The model under review builds one solid part; all positions refer to its coordinate system, in mm. A direction names the side the tool comes from. Coordinates: 2 decimals unless noted, no trailing zeros. Loops run counter-clockwise (first coordinate to the right, second up) from the corner with the lowest first, then second, coordinate; pieces in that order, holes last. Notation, with made-up numbers: (36, 81.25) - (69, 81.25) arc R28 ccw to (69, 107.25) - close; hole circle Ø8 at (58.5, -23.75). An arc over 180 degrees is marked (long way). Answer in a Markdown table with one row per item. Add a question column.
(1) We need section C-C on z = 6. Give the number of separate pieces and of enclosed holes in the cut face, plus the area to 3 significant figures.
(2) For line 1 along Y through (x, z) = (-15.5, 3.75); line 2 along Z through (x, y) = (-38, 23); line 3 along X through (y, z) = (8.5, 13.5), list the stretches that pass through material, from the lowest coordinate up.
(3) We need section A-A on x = 38.06. Write out the cut boundary in (y, z).
(4) Machinability: for faces 5 (the cylindrical face through (-15.676, 12.339, 3.549)), 6 (the flat face through (-2, 6, 4)), 7 (the flat face through (-22, 0, 8)), which of the approach directions +Z, -Z, +X, -X, +Y, -Y give a long, thin tool a straight path to every point of the face, cutting with its end or side? Answer none if there is none.
(5) We need section B-B on x = 4. Write out the cut boundary in (y, z), plus the area to 3 significant figures.
(6) We need section D-D on x = 26. Write out the cut boundary in (y, z).
(7) Mouldability with a two-part tool opening along Z and no side actions: class faces 1 (the flat face through (43.5, 23, 8)), 2 (the cylindrical face through (19, 15, 6)), 3 (the flat face through (19, 23, 8)), 4 (the flat face through (18, 17, 2)) as +Z half, -Z half, draft (parallel to the pull), parting line (faces both ways), or undercut.
(8) For P1, Ø2.5, axis at y = -9.5, z = 8, coming from the -X side; P2, Ø1.4, axis at x = 17.5, y = -16.5, coming from the +Z side; P3, Ø1, axis at x = 5, z = 12, coming from the +Y side, all flat-tipped, find the tip position at first contact; note any pin that passes through.
from build123d import *

# Parameters (mm, degrees)
F0_W      = 44
F0_H      = 41
F1_DEPTH  = 16
F2_R      = 1.35
F3_DEPTH  = 14
F6_DEPTH  = 9
F7_DEPTH  = 7
F8_R      = 1.35
F9_DEPTH  = 7.001
F11_R     = 3.2
F11_R_2   = 1.5
F11_R_3   = 2.625
F12_DEPTH = 10
F13_W     = 8
F13_H     = 3.8
F14_DEPTH = 12
F15_W     = 87
F15_H     = 16
F16_DEPTH = 6
F17_R     = 3.3
F18_DEPTH = 47.001
F19_R     = 3
F20_W     = 15
F20_H     = 12
F21_DEPTH = 3
F22_W     = 38
F22_H     = 11
F23_DEPTH = 7
F25_R     = 4
F26_DEPTH = 7


with BuildPart() as f1:
    # F0 (on Top) → F1 (new body)
    with BuildSketch(Plane.XY):
        Rectangle(F0_W, F0_H)
    extrude(amount=F1_DEPTH)

    # F2 (on face) → F3 (cut)
    with BuildSketch(Plane.XY.offset(16)):
        with BuildLine():
            Line((14, 16.5), (-14, 16.5))
            Line((-14, 16.5), (-14, -16.5))
            Line((-14, -16.5), (14, -16.5))
            ThreePointArc((14, -16.5), (15.1715728753, -13.6715728753), (18, -12.5))
            Line((18, -12.5), (18, 12.5))
            ThreePointArc((18, 12.5), (15.1715728753, 13.6715728753), (14, 16.5))
        make_face()
        with Locations((-18, 16.5)):
            Circle(F2_R)
        with Locations((18, 16.5)):
            Circle(F2_R)
        with Locations((-18, -16.5)):
            Circle(F2_R)
        with Locations((18, -16.5)):
            Circle(F2_R)
    extrude(amount=-F3_DEPTH, mode=Mode.SUBTRACT)

    # F5 (on face) → F6 (cut)
    with BuildSketch(Plane.XY.offset(16)):
        with BuildLine():
            ThreePointArc((-15.65, 16.5), (-16.5256357302, 14.6700409841), (-18.5, 14.2038074994))
            Line((-18.5, 14.2038074994), (-18.5, -14.2038074994))
            ThreePointArc((-18.5, -14.2038074994), (-16.5256357302, -14.6700409841), (-15.65, -16.5))
            Line((-15.65, -16.5), (-14, -16.5))
            Line((-14, -16.5), (-14, 16.5))
            Line((-14, 16.5), (-15.65, 16.5))
        make_face()
    extrude(amount=-F6_DEPTH, mode=Mode.SUBTRACT)

    # F4 (on Top) → F7 (join)
    with BuildSketch(Plane.XY):
        Polygon((-5, -1.15), (-5, -3.15), (2.5, -3.15), (2.5, 14.15), (-5, 14.15), (-5, 12.15), (-2, 12.15), (-2, -1.15), align=None)
    extrude(amount=F7_DEPTH)

    # F8 (on face) → F9 (cut, through all)
    with BuildSketch(Plane.XY.offset(7)):
        with Locations((-0.5, 5.5)):
            Circle(F8_R)
        with Locations((-15.5, 11)):
            Circle(F8_R)
        with Locations((-15.5, 0)):
            Circle(F8_R)
    extrude(amount=-F9_DEPTH, mode=Mode.SUBTRACT)

    # F11 (on face) → F12 (cut)
    with BuildSketch(Plane.YZ.offset(22)):
        with Locations((3, 6)):
            Circle(F11_R)
        with Locations((13.5, 6)):
            Circle(F11_R_2)
        with Locations((-10, 6)):
            Circle(F11_R_3)
    extrude(amount=-F12_DEPTH, mode=Mode.SUBTRACT)

    # F13 (on face) → F14 (cut)
    with BuildSketch(Plane.XY.offset(16)):
        with Locations((-18, 5.5)):
            Rectangle(F13_W, F13_H)
    extrude(amount=-F14_DEPTH, mode=Mode.SUBTRACT)

    # F15 (on face) → F16 (join)
    with BuildSketch(Plane(origin=(0, 20.5, 0), x_dir=(-1, 0, 0), z_dir=(0, 1, 0))):
        with Locations((0, 8)):
            Rectangle(F15_W, F15_H)
    extrude(amount=F16_DEPTH)

    # F17 (on face) → F18 (cut, through all)
    with BuildSketch(Plane(origin=(0, 26.5, 0), x_dir=(-1, 0, 0), z_dir=(0, 1, 0))):
        with Locations((38.06, 8)):
            Circle(F17_R)
        with Locations((-38.06, 8)):
            Circle(F17_R)
    extrude(amount=-F18_DEPTH, mode=Mode.SUBTRACT)

    # F19
    f19_edges = [f1.edges().sort_by_distance(p)[0] for p in [
        (43.5, 23.5, 16),
        (43.5, 23.5, 0),
        (-43.5, 23.5, 0),
        (-43.5, 23.5, 16),
    ]]
    fillet(f19_edges, radius=F19_R)

    # F20 (on face) → F21 (cut)
    with BuildSketch(Plane(origin=(18, 0, 0), x_dir=(0, -1, 0), z_dir=(-1, 0, 0))):
        with Locations((-3, 8)):
            Rectangle(F20_W, F20_H)
    extrude(amount=-F21_DEPTH, mode=Mode.SUBTRACT)

    # F22 (on face) → F23 (cut)
    with BuildSketch(Plane(origin=(0, 26.5, 0), x_dir=(-1, 0, 0), z_dir=(0, 1, 0))):
        with Locations((0, 8)):
            Rectangle(F22_W, F22_H)
    extrude(amount=-F23_DEPTH, mode=Mode.SUBTRACT)

    # F25 (on offset) → F26 (cut)
    with BuildSketch(Plane(origin=(13, 0, 0), x_dir=(0, -1, 0), z_dir=(-1, 0, 0))):
        with Locations((10, 6)):
            Circle(F25_R)
    extrude(amount=-F26_DEPTH, mode=Mode.SUBTRACT)


solid = f1.part
Outcome:
| question | item | result |
|---|---|---|
| 1 | separate pieces | 7 |
| 1 | enclosed holes | 7 |
| 1 | area | 886 mm² |
| 2 | line 1 | -20.5 to -1.35, 1.35 to 9.65, 12.35 to 19.5 |
| 2 | line 2 | 0 to 4.7, 11.3 to 16 |
| 2 | line 3 | -22 to -18.5, 21 to 22 |
| 3 | outline | (20.5, 0) - (26.5, 0) - (26.5, 4.7) - (20.5, 4.7) - close; (20.5, 11.3) - (26.5, 11.3) - (26.5, 16) - (20.5, 16) - close |
| 4 | face 5 | +Z, -Z |
| 4 | face 6 | +Z |
| 4 | face 7 | +Z, -Z, -X, -Y |
| 5 | outline | (-20.5, 0) - (26.5, 0) - (26.5, 2.5) - (19.5, 2.5) - (19.5, 13.5) - (26.5, 13.5) - (26.5, 16) - (16.5, 16) - (16.5, 2) - (-16.5, 2) - (-16.5, 16) - (-20.5, 16) - close |
| 5 | area | 213 mm² |
| 6 | outline | (20.5, 0) - (26.5, 0) - (26.5, 16) - (20.5, 16) - close |
| 7 | face 1 | draft |
| 7 | face 2 | undercut |
| 7 | face 3 | undercut |
| 7 | face 4 | +Z half |
| 8 | P1 | x = -22 |
| 8 | P2 | z = 2 |
| 8 | P3 | y = 19.5 |
